```python
from build123d import *

# Parameters (mm, degrees)
SKETCH1_R           = 19.5
SKETCH1_R_2         = 17.5
BOSS_EXTRUDE1_DEPTH = 3.5
SKETCH2_R           = 7
BOSS_EXTRUDE2_DEPTH = 2
BOSS_EXTRUDE3_DEPTH = 3.5
SKETCH8_R           = 3.5
CUT_EXTRUDE1_DEPTH  = 28.649593125


with BuildPart() as part:
    # Sketch1 → Boss-Extrude1 (new body)
    with BuildSketch(Plane(origin=(0, 0, 0), x_dir=(1, 0, 0), z_dir=(0, 1, 0))):
        with Locations(Location((0, 0, 0), (0, 0, 270))):
            Circle(SKETCH1_R)
        with Locations(Location((0, 0, 0), (0, 0, 270))):
            Circle(SKETCH1_R_2, mode=Mode.SUBTRACT)
    extrude(amount=BOSS_EXTRUDE1_DEPTH)



with BuildPart() as body_2:
    # Sketch2 → Boss-Extrude2 (new body)
    with BuildSketch(Plane(origin=(0, 0, 0), x_dir=(1, 0, 0), z_dir=(0, 1, 0))):
        with Locations(Location((0, 0, 0), (0, 0, 270))):
            Circle(SKETCH2_R)
    extrude(amount=BOSS_EXTRUDE2_DEPTH)


with BuildPart() as part_1:
    add(part.part)

    add(body_2.part)  # Boss-Extrude3 merges body 2
    # Sketch4 → Boss-Extrude3 (add)
    with BuildSketch(Plane(origin=(0, 0, 0), x_dir=(1, 0, 0), z_dir=(0, 1, 0))):
        with BuildLine():
            Line((0.76143589, 6.958463579), (1.903589725, 17.396158948))
            ThreePointArc((1.903589725, 17.396158948), (3.038843109, 17.234135678), (4.161047559, 16.998108224))
            Line((4.161047559, 16.998108224), (1.664419024, 6.79924329))
            ThreePointArc((1.664419024, 6.79924329), (1.215537244, 6.893654271), (0.76143589, 6.958463579))
        make_face()
        with BuildLine():
            Line((3.095450398, 6.278390465), (7.738625995, 15.695976163))
            ThreePointArc((7.738625995, 15.695976163), (8.75, 15.155444566), (9.723801097, 14.549834783))
            Line((9.723801097, 14.549834783), (3.889520439, 5.819933913))
            ThreePointArc((3.889520439, 5.819933913), (3.5, 6.062177826), (3.095450398, 6.278390465))
        make_face()
        with BuildLine():
            Line((5.056107904, 4.841050802), (12.640269759, 12.102627005))
            ThreePointArc((12.640269759, 12.102627005), (13.405777755, 11.24878317), (14.113720715, 10.346636535))
            Line((14.113720715, 10.346636535), (5.645488286, 4.138654614))
            ThreePointArc((5.645488286, 4.138654614), (5.362311102, 4.499513268), (5.056107904, 4.841050802))
        make_face()
        with BuildLine():
            Line((6.406924176, 2.819808966), (16.01731044, 7.049522414))
            ThreePointArc((16.01731044, 7.049522414), (16.444620864, 5.985352508), (16.801317318, 4.89548122))
            Line((16.801317318, 4.89548122), (6.720526927, 1.958192488))
            ThreePointArc((6.720526927, 1.958192488), (6.577848346, 2.394141003), (6.406924176, 2.819808966))
        make_face()
        with BuildLine():
            Line((6.984970837, 0.458456552), (17.462427092, 1.14614138))
            ThreePointArc((17.462427092, 1.14614138), (17.5, 0), (17.462427092, -1.14614138))
            Line((17.462427092, -1.14614138), (6.984970837, -0.458456552))
            ThreePointArc((6.984970837, -0.458456552), (7, 0), (6.984970837, 0.458456552))
        make_face()
        with BuildLine():
            Line((6.720526927, -1.958192488), (16.801317318, -4.89548122))
            ThreePointArc((16.801317318, -4.89548122), (16.444620864, -5.985352508), (16.01731044, -7.049522414))
            Line((16.01731044, -7.049522414), (6.406924176, -2.819808966))
            ThreePointArc((6.406924176, -2.819808966), (6.577848346, -2.394141003), (6.720526927, -1.958192488))
        make_face()
        with BuildLine():
            Line((5.645488286, -4.138654614), (14.113720715, -10.346636535))
            ThreePointArc((14.113720715, -10.346636535), (13.405777755, -11.24878317), (12.640269759, -12.102627005))
            Line((12.640269759, -12.102627005), (5.056107904, -4.841050802))
            ThreePointArc((5.056107904, -4.841050802), (5.362311102, -4.499513268), (5.645488286, -4.138654614))
        make_face()
        with BuildLine():
            Line((3.889520439, -5.819933913), (9.723801097, -14.549834783))
            ThreePointArc((9.723801097, -14.549834783), (8.75, -15.155444566), (7.738625995, -15.695976163))
            Line((7.738625995, -15.695976163), (3.095450398, -6.278390465))
            ThreePointArc((3.095450398, -6.278390465), (3.5, -6.062177826), (3.889520439, -5.819933913))
        make_face()
        with BuildLine():
            Line((1.664419024, -6.79924329), (4.161047559, -16.998108224))
            ThreePointArc((4.161047559, -16.998108224), (3.038843109, -17.234135678), (1.903589725, -17.396158948))
            Line((1.903589725, -17.396158948), (0.76143589, -6.958463579))
            ThreePointArc((0.76143589, -6.958463579), (1.215537244, -6.893654271), (1.664419024, -6.79924329))
        make_face()
        with BuildLine():
            Line((-0.76143589, -6.958463579), (-1.903589725, -17.396158948))
            ThreePointArc((-1.903589725, -17.396158948), (-3.038843109, -17.234135678), (-4.161047559, -16.998108224))
            Line((-4.161047559, -16.998108224), (-1.664419024, -6.79924329))
            ThreePointArc((-1.664419024, -6.79924329), (-1.215537244, -6.893654271), (-0.76143589, -6.958463579))
        make_face()
        with BuildLine():
            Line((-3.095450398, -6.278390465), (-7.738625995, -15.695976163))
            ThreePointArc((-7.738625995, -15.695976163), (-8.75, -15.155444566), (-9.723801097, -14.549834783))
            Line((-9.723801097, -14.549834783), (-3.889520439, -5.819933913))
            ThreePointArc((-3.889520439, -5.819933913), (-3.5, -6.062177826), (-3.095450398, -6.278390465))
        make_face()
        with BuildLine():
            Line((-5.056107904, -4.841050802), (-12.640269759, -12.102627005))
            ThreePointArc((-12.640269759, -12.102627005), (-13.405777755, -11.24878317), (-14.113720715, -10.346636535))
            Line((-14.113720715, -10.346636535), (-5.645488286, -4.138654614))
            ThreePointArc((-5.645488286, -4.138654614), (-5.362311102, -4.499513268), (-5.056107904, -4.841050802))
        make_face()
        with BuildLine():
            Line((-6.406924176, -2.819808966), (-16.01731044, -7.049522414))
            ThreePointArc((-16.01731044, -7.049522414), (-16.444620864, -5.985352508), (-16.801317318, -4.89548122))
            Line((-16.801317318, -4.89548122), (-6.720526927, -1.958192488))
            ThreePointArc((-6.720526927, -1.958192488), (-6.577848346, -2.394141003), (-6.406924176, -2.819808966))
        make_face()
        with BuildLine():
            Line((-6.984970837, -0.458456552), (-17.462427092, -1.14614138))
            ThreePointArc((-17.462427092, -1.14614138), (-17.5, 0), (-17.462427092, 1.14614138))
            Line((-17.462427092, 1.14614138), (-6.984970837, 0.458456552))
            ThreePointArc((-6.984970837, 0.458456552), (-7, 0), (-6.984970837, -0.458456552))
        make_face()
        with BuildLine():
            Line((-6.720526927, 1.958192488), (-16.801317318, 4.89548122))
            ThreePointArc((-16.801317318, 4.89548122), (-16.444620864, 5.985352508), (-16.01731044, 7.049522414))
            Line((-16.01731044, 7.049522414), (-6.406924176, 2.819808966))
            ThreePointArc((-6.406924176, 2.819808966), (-6.577848346, 2.394141003), (-6.720526927, 1.958192488))
        make_face()
        with BuildLine():
            Line((-5.645488286, 4.138654614), (-14.113720715, 10.346636535))
            ThreePointArc((-14.113720715, 10.346636535), (-13.405777755, 11.24878317), (-12.640269759, 12.102627005))
            Line((-12.640269759, 12.102627005), (-5.056107904, 4.841050802))
            ThreePointArc((-5.056107904, 4.841050802), (-5.362311102, 4.499513268), (-5.645488286, 4.138654614))
        make_face()
        with BuildLine():
            Line((-3.889520439, 5.819933913), (-9.723801097, 14.549834783))
            ThreePointArc((-9.723801097, 14.549834783), (-8.75, 15.155444566), (-7.738625995, 15.695976163))
            Line((-7.738625995, 15.695976163), (-3.095450398, 6.278390465))
            ThreePointArc((-3.095450398, 6.278390465), (-3.5, 6.062177826), (-3.889520439, 5.819933913))
        make_face()
        with BuildLine():
            Line((-1.664419024, 6.79924329), (-4.161047559, 16.998108224))
            ThreePointArc((-4.161047559, 16.998108224), (-3.038843109, 17.234135678), (-1.903589725, 17.396158948))
            Line((-1.903589725, 17.396158948), (-0.76143589, 6.958463579))
            ThreePointArc((-0.76143589, 6.958463579), (-1.215537244, 6.893654271), (-1.664419024, 6.79924329))
        make_face()
    extrude(amount=BOSS_EXTRUDE3_DEPTH)

    # Sketch7 → Cut-Revolve1 (revolve, cut)
    with BuildSketch(Plane.XY):
        Polygon((7, 2), (17.5, 3.5), (7, 3.5), align=None)
    revolve(axis=Axis((0, -983.4456259, 0), (0, 1, 0)), mode=Mode.SUBTRACT)

    # Sketch8 → Cut-Extrude1 (cut, through all)
    with BuildSketch(Plane(origin=(0, 2, 0), x_dir=(1, 0, 0), z_dir=(0, 1, 0))):
        with Locations(Location((0, 0, 0), (0, 0, 270))):
            Circle(SKETCH8_R)
    extrude(amount=-CUT_EXTRUDE1_DEPTH, mode=Mode.SUBTRACT)


solid = part_1.part
```
Source: CAD feature listing. Evaluate the final solid. Frame: model axes, mm. A direction names the side the tool comes from. Give positions to 0.01 mm unless a question says otherwise; leave off trailing zeros. Write each loop counter-clockwise with the first axis right and the second up, starting at its lowest first coordinate (ties: lowest second). Pieces come first, ordered by that corner, then holes.
1. Section query A-A (z = 0). Return the cut outline in (x, y), then the cut area to 4 significant figures.
2. Section query C-C (y = 0.5). Count the separate pieces of the cut face and the enclosed holes in it, then the cut area to 3 significant figures.
3. Pull-direction query (Z, two-part tool) for faces 3 (the face through (-1.34, 1.34, -12.25)), 4 (the face through (-8.9, 1.34, -8.52)); classes: +Z half, -Z half, draft (parallel to the pull), parting line (faces both ways), or undercut.
4. Section query B-B (x = 0). Return the cut outline in (y, z), then the cut area to 3 significant figures.
5. First-contact query: pin 1 (1 mm diameter, centred on y = 1, z = 6, fed in from -X); pin 2 (11 mm diameter, centred on x = 1, z = 0.5, fed in from +Y); pin 3 (1.5 mm diameter, centred on x = -3, z = 7, fed in from +Y); pin 4 (5.5 mm diameter, centred on x = 0, z = 0, fed in from -Y). Flat tips, straight axial feed; report the tip coordinate or a pass-through.
6. Access query for faces 1 (the face through (-11.58, 2.76, 4.2)), 2 (the face through (-11.145, 1.337, 4.905)). Directions: +Z, -Z, +X, -X, +Y, -Y. A direction counts if a zero-diameter tool reaches every point of the face in a straight line with its end or side. Return the directions, or none.
7. Material intervals for line 1 along X through (y, z) = (1.2, 0); line 2 along X through (y, z) = (0.55, 10.5); line 3 along X through (y, z) = (1.9, -11.5), sorted ascending.
Output values:
1. outline: (-19.5, 0) - (-3.5, 0) - (-3.5, 2) - (-7, 2) - (-17.5, 3.5) - (-19.5, 3.5) - close; (3.5, 0) - (19.5, 0) - (19.5, 3.5) - (17.5, 3.5) - (7, 2) - (3.5, 2) - close
1. area: 85.75 mm2
2. separate pieces: 1
2. enclosed holes: 19
2. area: 651 mm2
3. face 3: undercut
3. face 4: undercut
4. outline: (0, -19.5) - (3.5, -19.5) - (3.5, -17.5) - (0, -17.5) - close; (0, -7) - (2, -7) - (2, -3.5) - (0, -3.5) - close; (0, 3.5) - (2, 3.5) - (2, 7) - (0, 7) - close; (0, 17.5) - (3.5, 17.5) - (3.5, 19.5) - (0, 19.5) - close
4. area: 28.0 mm2
5. pin 1: stops at x = -18.71
5. pin 2: stops at y = 2
5. pin 3: stops at y = 2.18
5. pin 4: passes through
6. face 1: +Y
6. face 2: +Y, -Y
7. line 1: x = -19.5 to -3.5, 3.5 to 19.5
7. line 2: x = -16.43 to -10.97, -7.02 to -5.18, -2.57 to -1.15, 1.15 to 2.57, 5.18 to 7.02, 10.97 to 16.43
7. line 3: x = -15.75 to -12.01, -7.69 to -5.67, -2.82 to -1.26, 1.26 to 2.82, 5.67 to 7.69, 12.01 to 15.75
